Here's how the part is built. I have some questions about the finished solid (model axes, mm). Round coordinates to 2 decimals unless told otherwise and drop trailing zeros. Write each loop counter-clockwise with the first axis right and the second up, starting at its lowest first coordinate (ties: lowest second). Pieces come first, ordered by that corner, then holes. Notation, with made-up numbers: (38, 41.25) -> (45, 41.25) arc R19 ccw to (45, 74.25) -> close; hole circle Ø1 at (66, 19). An arc over 180 degrees is marked (long way). Answer in a Markdown table with one row per item.
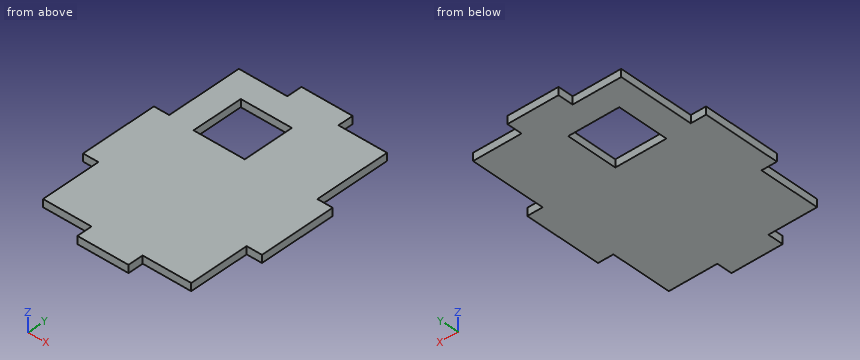
from build123d import *

# Parameters (mm, degrees)
ESQUISSE1_W             = 70
ESQUISSE1_H             = 95
BOSS_EXTRU_1_DEPTH      = 3
ESQUISSE2_W             = 20
ESQUISSE2_H             = 20
ENL_V_MAT_EXTRU_1_DEPTH = 119.042365276


with BuildPart() as part:
    # Esquisse1 → Boss.-Extru.1 (new body)
    with BuildSketch(Plane.XY):
        with Locations((-35, 47.5)):
            Rectangle(ESQUISSE1_W, ESQUISSE1_H)
    extrude(amount=BOSS_EXTRU_1_DEPTH)

    # Esquisse2 → Enlèv. mat.-Extru.1 (cut, through all)
    with BuildSketch(Plane(origin=(0, 0, 0), x_dir=(-1, 0, 0), z_dir=(0, 0, -1))):
        Polygon((0, 95), (25, 95), (25, 89), (6, 89), (6, 59.5), (0, 59.5), align=None)
        Polygon((70, 95), (45, 95), (45, 89), (64, 89), (64, 59.5), (70, 59.5), align=None)
        Polygon((0, 0), (25, 0), (25, 6), (6, 6), (6, 29.5), (0, 29.5), align=None)
        Polygon((45, 0), (70, 0), (70, 29.5), (64, 29.5), (64, 6), (45, 6), align=None)
        with Locations((44, 69)):
            Rectangle(ESQUISSE2_W, ESQUISSE2_H)
    extrude(amount=-ENL_V_MAT_EXTRU_1_DEPTH, mode=Mode.SUBTRACT)


solid = part.part
1) I want a section at C-C, the plane y = 80. List the corners of the cut face in (x, z) for me, and give its area (3 significant figures).
Response:
| item | result |
|---|---|
| outline | (-64, 0) -> (-6, 0) -> (-6, 3) -> (-64, 3) -> close |
| area | 174 mm^2 |
2) I want a section at A-A, the plane x = -36.5. List the corners of the cut face in (y, z) for me, and give its area (3 significant figures).
Response:
| item | result |
|---|---|
| outline | (0, 0) -> (59, 0) -> (59, 3) -> (0, 3) -> close; (79, 0) -> (95, 0) -> (95, 3) -> (79, 3) -> close |
| area | 225 mm^2 |
3) For pin 1 (1.5 mm diameter, centred on x = -19, z = 1.5, fed in from -Y); pin 2 (1.5 mm diameter, centred on y = 73.5, z = 2, fed in from +X); pin 3 (1.5 mm diameter, centred on y = 74.5, z = 2, fed in from -X); pin 4 (1.5 mm diameter, centred on x = -42.5, z = 1.5, fed in from -Y), each with a flat end and sliding along its axis, tell me the tip position at first contact or that it passes through.
Response:
| item | result |
|---|---|
| pin 1 | stops at y = 6 |
| pin 2 | stops at x = -6 |
| pin 3 | stops at x = -64 |
| pin 4 | stops at y = 0 |
4) I want a section at D-D, the plane x = -8. List the corners of the cut face in (y, z) for me, and give its area (3 significant figures).
Response:
| item | result |
|---|---|
| outline | (6, 0) -> (89, 0) -> (89, 3) -> (6, 3) -> close |
| area | 249 mm^2 |
5) I want a section at B-B, the plane z = 1.45. List the corners of the cut face in (x, y) for me.
Response:
| item | result |
|---|---|
| outline | (-70, 29.5) -> (-64, 29.5) -> (-64, 6) -> (-45, 6) -> (-45, 0) -> (-25, 0) -> (-25, 6) -> (-6, 6) -> (-6, 29.5) -> (0, 29.5) -> (0, 59.5) -> (-6, 59.5) -> (-6, 89) -> (-25, 89) -> (-25, 95) -> (-45, 95) -> (-45, 89) -> (-64, 89) -> (-64, 59.5) -> (-70, 59.5) -> close; hole (-54, 59) -> (-34, 59) -> (-34, 79) -> (-54, 79) -> close |
6) I need wall thicknesses on line 1 (X direction, y = 66.5, z = 1); line 2 (Y direction, x = -47.5, z = 0.85); line 3 (X direction, y = 82, z = 0.35). Which ranges of each line are inside material? Lowest first, please. Write a range as [from, to].
Response:
| item | result |
|---|---|
| line 1 | x = [-64, -54], [-34, -6] |
| line 2 | y = [6, 59], [79, 89] |
| line 3 | x = [-64, -6] |
